Verification items for the finished model (mm, model axes). Coordinates: 2 decimals unless noted, no trailing zeros. Order: outer loops, then holes, each group sorted by start corner. A loop starts at its lowest first (then second) coordinate and runs counter-clockwise, first axis right, second up. Notation, with made-up numbers: M -7.5,-21 L 32.5,-21 A16 cw 32.5,-4 Z; hole C -13.75,58.25 d10. An arc over 180 degrees is marked long. Answer as a JSON object with one key per item and string values. Group by question number.
(1) Material ranges on line 1 (X direction, y = 6, z = 1.45); line 2 (Y direction, x = -121.5, z = 1.1); line 3 (Y direction, x = -122.5, z = 0.45), recorded low to high.
(2) Cross-section at C-C (y = 27). Enter the section's corners in (x, z), plus the area to 3 significant figures.
(3) Cross-section at B-B (x = -74). Enter the section's corners in (y, z), plus the area to 3 significant figures.
(4) Gauge pin test, flat end, axial feed: pin 1 Ø0.8 at (x, z) = (-117.5, 1) entering from +Y. Record the tip position at first contact, or that the pin passes through.
(5) Cross-section at A-A (z = 0.6). Enter the section's corners in (x, y).
(6) Mould release check, pull along X, two halves, no side actions. Record for faces 1 (the face through (-76, 16, 1.588)), 2 (the face through (-73.579, 32.395, 0.783)), 3 (the face through (-131.51, 8.03, 0.78)): released by +X, released by -X, zero draft, split by the parting line, or undercut.
from build123d import *

# Parameters (mm, degrees)
ESQUISSE1_R        = 1.59
BOSS_EXTRU_1_DEPTH = 1.5875
CONG_1_R           = 2


with BuildPart() as part:
    # Esquisse1 → Boss.-Extru.1 (new body)
    with BuildSketch(Plane.XY):
        Polygon((-149.248115566, 40), (-149.248115566, 0), (0, 0), (0, 25), align=None)
        with Locations((-130.248115566, 9)):
            Circle(ESQUISSE1_R, mode=Mode.SUBTRACT)
        with Locations((-105.258115566, 9)):
            Circle(ESQUISSE1_R, mode=Mode.SUBTRACT)
        Polygon((-127.253115566, 12.25), (-108.253115566, 12.25), (-109.753115566, 5.75), (-125.753115566, 5.75), align=None, mode=Mode.SUBTRACT)
    extrude(amount=BOSS_EXTRU_1_DEPTH)

    # Congé1
    cong_1_edges = [part.edges().sort_by_distance(p)[0] for p in [
        (-127.253115566, 12.25, 0.79375),
        (-125.753115566, 5.75, 0.79375),
        (-109.753115566, 5.75, 0.79375),
        (-108.253115566, 12.25, 0.79375),
    ]]
    fillet(cong_1_edges, radius=CONG_1_R)


solid = part.part
Taken from the geometry:
{
 "1": {"line 1": "x = -149.25 to -125.13, -110.38 to 0", "line 2": "y = 0 to 5.75, 12.25 to 37.21", "line 3": "y = 0 to 5.75, 12.25 to 37.31"},
 "2": {"outline": "M -149.25,0 L -19.9,0 L -19.9,1.59 L -149.25,1.59 Z", "area": "205 mm²"},
 "3": {"outline": "M 0,0 L 32.44,0 L 32.44,1.59 L 0,1.59 Z", "area": "51.5 mm²"},
 "4": {"pin 1": "stops at y = 36.85"},
 "5": {"outline": "M -149.25,0 L 0,0 L 0,25 L -149.25,40 Z; hole C -130.25,9 d3.18; hole M -126.69,9.8 L -126.11,7.3 A2 ccw -124.16,5.75 L -111.34,5.75 A2 ccw -109.4,7.3 L -108.82,9.8 A2 ccw -110.77,12.25 L -124.74,12.25 A2 ccw Z; hole C -105.26,9 d3.18"},
 "6": {"face 1": "zero draft", "face 2": "released by +X", "face 3": "undercut"}
}
